The model under review builds one solid part; all positions refer to its coordinate system, in mm. A direction names the side the tool comes from. Give positions to 0.01 mm unless a question says otherwise; leave off trailing zeros. Write each loop counter-clockwise with the first axis right and the second up, starting at its lowest first coordinate (ties: lowest second). Pieces come first, ordered by that corner, then holes. Notation, with made-up numbers: (43.25, -31.75) -> (74.25, -31.75) arc R27 ccw to (74.25, -4.75) -> close; hole circle Ø2 at (12, -26). An arc over 180 degrees is marked (long way). Use CSV: the item, a comma, the result in double quotes.
```python
from build123d import *

# Parameters (mm, degrees)
BOSS_EXTRU_1_DEPTH                             = 15
ESQUISSE2_R                                    = 1.2
ENL_V_MAT_EXTRU_1_DEPTH                        = 26.243811123
ESQUISSE3_R                                    = 0.75
ENL_V_MAT_EXTRU_2_DEPTH                        = 20.006577809
ESQUISSE4_R                                    = 1.2
ENL_V_MAT_EXTRU_3_DEPTH                        = 34.470135942
BOSS_EXTRU_2_START                             = 2.3
ESQUISSE5_W                                    = 5.3
ESQUISSE5_H                                    = 9.6
ESQUISSE5_R                                    = 0.75
BOSS_EXTRU_2_DEPTH                             = 2.3
FRAISAGE_POUR_VIS_T_TE_FRAIS_E_M31_D           = 3.2
FRAISAGE_POUR_VIS_T_TE_FRAIS_E_M31_CSINK_D     = 6.3
FRAISAGE_POUR_VIS_T_TE_FRAIS_E_M31_CSINK_ANGLE = 90
ENL_V_MAT_EXTRU_4_DEPTH                        = 2.3
ESQUISSE9_R                                    = 1.2
ENL_V_MAT_EXTRU_5_DEPTH                        = 20.006577853


with BuildPart() as part:
    # Esquisse1 → Boss.-Extru.1 (new, symmetric)
    with BuildSketch(Plane(origin=(0, 0, 0), x_dir=(0, 0, -1), z_dir=(1, 0, 0))):
        Polygon((-12.5, -4.8), (-12.5, -8), (0, -8), (0, 8), (-12.5, 8), (-12.5, 4.8), (-8.5, 4.8), (-8.5, -4.8), align=None)
    extrude(amount=BOSS_EXTRU_1_DEPTH, both=True)

    # Esquisse2 → Enlèv. mat.-Extru.1 (cut, through all)
    with BuildSketch(Plane(origin=(0, 8, 0), x_dir=(1, 0, 0), z_dir=(0, 1, 0))):
        with Locations(Location((-7.5, -4, 0), (0, 0, 270))):
            Circle(ESQUISSE2_R)
        with Locations(Location((7.5, -4, 0), (0, 0, 90))):
            Circle(ESQUISSE2_R)
        with Locations(Location((0, -4, 0), (0, 0, 270))):
            Circle(ESQUISSE2_R)
    extrude(amount=-ENL_V_MAT_EXTRU_1_DEPTH, mode=Mode.SUBTRACT)

    # Esquisse3 → Enlèv. mat.-Extru.2 (cut, through all)
    with BuildSketch(Plane.XY.offset(8.5)):
        with Locations((-12, 0)):
            Circle(ESQUISSE3_R)
    extrude(amount=-ENL_V_MAT_EXTRU_2_DEPTH, mode=Mode.SUBTRACT)

    # Esquisse4 → Enlèv. mat.-Extru.3 (cut, through all)
    with BuildSketch(Plane(origin=(15, 0, 0), x_dir=(0, 0, -1), z_dir=(1, 0, 0))):
        with Locations((-4, -4.5)):
            Circle(ESQUISSE4_R)
        with Locations(Location((-4, 4.5, 0), (0, 0, 180))):
            Circle(ESQUISSE4_R)
    extrude(amount=-ENL_V_MAT_EXTRU_3_DEPTH, mode=Mode.SUBTRACT)

    # Esquisse5 → Boss.-Extru.2 (add)
    with BuildSketch(Plane.XY.offset(8.5).offset(BOSS_EXTRU_2_START)):
        with Locations((-12.35, 0)):
            Rectangle(ESQUISSE5_W, ESQUISSE5_H)
        with Locations((-12, 0)):
            Circle(ESQUISSE5_R, mode=Mode.SUBTRACT)
    extrude(amount=-BOSS_EXTRU_2_DEPTH)

    # Fraisage pour vis à tête fraisée M31 (through all)
    with Locations(Plane.XY.offset(8.5)):
        with Locations((0, 0)):
            CounterSinkHole(FRAISAGE_POUR_VIS_T_TE_FRAIS_E_M31_D / 2, FRAISAGE_POUR_VIS_T_TE_FRAIS_E_M31_CSINK_D / 2, counter_sink_angle=FRAISAGE_POUR_VIS_T_TE_FRAIS_E_M31_CSINK_ANGLE)

    # Esquisse8 → Enlèv. mat.-Extru.4 (cut)
    with BuildSketch(Plane(origin=(0, 0, 0), x_dir=(-1, 0, 0), z_dir=(0, 0, -1))):
        Polygon((14.8, 1.616580754), (12, 3.233161507), (9.2, 1.616580754), (9.2, -1.616580754), (12, -3.233161507), (14.8, -1.616580754), align=None)
    extrude(amount=-ENL_V_MAT_EXTRU_4_DEPTH, mode=Mode.SUBTRACT)

    # Esquisse9 → Enlèv. mat.-Extru.5 (cut, through all)
    with BuildSketch(Plane.XY.offset(8.5)):
        with Locations((5, 0)):
            Circle(ESQUISSE9_R)
    extrude(amount=-ENL_V_MAT_EXTRU_5_DEPTH, mode=Mode.SUBTRACT)


solid = part.part
```
Q1. Consider section D-D (z = 5.5). Write out the cut boundary in (x, y), then the cut area to 3 significant figures.
Derived:
outline,"(-15, -8) -> (15, -8) -> (15, 8) -> (-15, 8) -> close; hole circle Ø1.5 at (-12, 0); hole circle Ø3.2 at (0, 0); hole circle Ø2.4 at (5, 0)"
area,"466 mm2"
Q2. Machinability: for faces 1 (the flat face through (-13, 0, 10.8)), 2 (the cylindrical face through (11.302, -4.14, 2.855)), 3 (the flat face through (0, 4.8, 11)), which of the approach directions +Z, -Z, +X, -X, +Y, -Y give a long, thin tool a straight path to every point of the face, cutting with its end or side? Answer none if there is none.
Derived:
face 1,"+Z, +X, -X"
face 2,"+X, -X"
face 3,"+Z, +X"
Q3. The part is to be moulded in two halves that separate along Z. For faces 4 (the cylindrical face through (-7.14, 0.063, 5.145)), 5 (the cylindrical face through (3.8, 0.05, 4.31)), 6 (the flat face through (0, -6, 12.5)), say which applies: pulls with the +Z half, pulls with the -Z half, needs draft (parallel to the pull), parting line crosses it, or undercut.
Derived:
face 4,"undercut"
face 5,"needs draft"
face 6,"pulls with the +Z half"
Q4. Consider section A-A (y = 0). Write out the cut boundary in (x, z).
Derived:
outline,"(-15, 0) -> (-14.8, 0) -> (-14.8, 2.3) -> (-12.75, 2.3) -> (-12.75, 10.8) -> (-15, 10.8) -> close; (-11.25, 2.3) -> (-9.2, 2.3) -> (-9.2, 0) -> (-1.6, 0) -> (-1.6, 6.95) -> (-3.15, 8.5) -> (-9.7, 8.5) -> (-9.7, 10.8) -> (-11.25, 10.8) -> close; (1.6, 0) -> (3.8, 0) -> (3.8, 8.5) -> (3.15, 8.5) -> (1.6, 6.95) -> close; (6.2, 0) -> (15, 0) -> (15, 8.5) -> (6.2, 8.5) -> close; hole circle Ø2.4 at (-7.5, 4); hole circle Ø2.4 at (7.5, 4)"
Q5. Consider section C-C (x = 5). Write out the cut boundary in (y, z).
Derived:
outline,"(-8, 0) -> (-1.2, 0) -> (-1.2, 8.5) -> (-4.8, 8.5) -> (-4.8, 12.5) -> (-8, 12.5) -> close; (1.2, 0) -> (8, 0) -> (8, 12.5) -> (4.8, 12.5) -> (4.8, 8.5) -> (1.2, 8.5) -> close; hole circle Ø2.4 at (-4.5, 4); hole circle Ø2.4 at (4.5, 4)"
Q6. Consider section B-B (z = 11.5). Write out the cut boundary in (x, y), then the cut area to 3 significant figures.
Derived:
outline,"(-15, -8) -> (15, -8) -> (15, -4.8) -> (-15, -4.8) -> close; (-15, 4.8) -> (15, 4.8) -> (15, 8) -> (-15, 8) -> close"
area,"192 mm2"
Q7. Insertion check: pin 1 (4 mm diameter, centred on x = 0, z = 4, fed in from +Y); pin 2 (3 mm diameter, centred on x = -11.5, y = 1, fed in from -Z). Each pin has a flat end and moves straight along its axis. Give the tip position at first contact, or say it passes through.
Derived:
pin 1,"stops at y = 8"
pin 2,"stops at z = 2.3"
Q8. To check wall thickness, follow probe 1 along Y at (x, z) = (-5, 4); probe 2 along X at (y, z) = (7.3, 4); probe 3 along Z at (x, y) = (7.5, 7.35). State the ranges of each line that lie inside material, in increasing order.
Derived:
probe 1,"y = -8 to -5.7, -3.3 to 3.3, 5.7 to 8"
probe 2,"x = -15 to -8.7, -6.3 to -1.2, 1.2 to 6.3, 8.7 to 15"
probe 3,"z = 0 to 2.8, 5.2 to 12.5"
